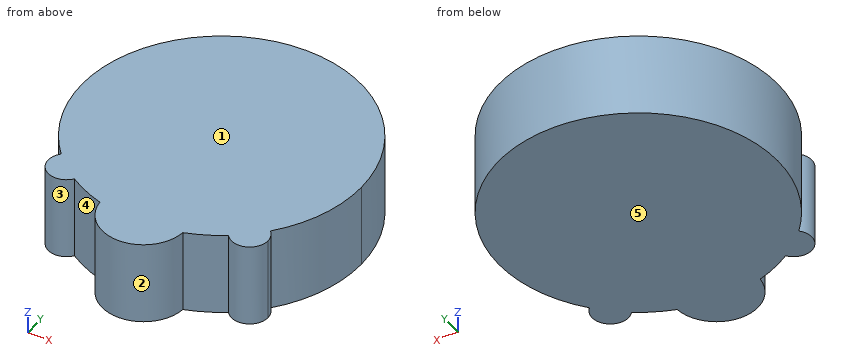
```python
from build123d import *

# Parameters (mm, degrees)
F1_DEPTH = 25


with BuildPart() as f1:
    # F0 (on Top) → F1 (new body)
    with BuildSketch(Plane.XY):
        with BuildLine():
            ThreePointArc((31.4123807864, -27.8794249104), (39.2639783582, -14.9110698304), (42, 0))
            ThreePointArc((42, 0), (-14.9110698304, 39.2639783582), (-31.4123807864, -27.8794249104))
            ThreePointArc((-31.4123807864, -27.8794249104), (-25.4105137384, -26.6574416615), (-22, -31.7450783587))
            ThreePointArc((-22, -31.7450783587), (-22.2864690998, -33.4969617889), (-23.1160347465, -35.066350503))
            ThreePointArc((-23.1160347465, -35.066350503), (-17.9613012827, -37.9656641748), (-12.4504239602, -40.1121794872))
            ThreePointArc((-12.4504239602, -40.1121794872), (-0.5566419395, -26.5124001605), (12.5, -39))
            ThreePointArc((12.5, -39), (12.4875998395, -39.5566419395), (12.4504239602, -40.1121794872))
            ThreePointArc((12.4504239602, -40.1121794872), (17.9613012827, -37.9656641748), (23.1160347465, -35.066350503))
            ThreePointArc((23.1160347465, -35.066350503), (23.8988095238, -27.5879847641), (31.4123807864, -27.8794249104))
        make_face()
        with BuildLine():
            ThreePointArc((-22, -31.7450783587), (-25.4105137384, -26.6574416615), (-31.4123807864, -27.8794249104))
            ThreePointArc((-31.4123807864, -27.8794249104), (-27.5, -31.7450783587), (-23.1160347465, -35.066350503))
            ThreePointArc((-23.1160347465, -35.066350503), (-22.2864690998, -33.4969617889), (-22, -31.7450783587))
        make_face()
        with BuildLine():
            ThreePointArc((-23.1160347465, -35.066350503), (-27.5, -31.7450783587), (-31.4123807864, -27.8794249104))
            ThreePointArc((-31.4123807864, -27.8794249104), (-31.1011904762, -35.9021719533), (-23.1160347465, -35.066350503))
        make_face()
        with BuildLine():
            ThreePointArc((33, -31.7450783587), (32.5876366972, -29.6555920971), (31.4123807864, -27.8794249104))
            ThreePointArc((31.4123807864, -27.8794249104), (27.5, -31.7450783587), (23.1160347465, -35.066350503))
            ThreePointArc((23.1160347465, -35.066350503), (29.2518834302, -36.9586092589), (33, -31.7450783587))
        make_face()
        with BuildLine():
            ThreePointArc((23.1160347465, -35.066350503), (27.5, -31.7450783587), (31.4123807864, -27.8794249104))
            ThreePointArc((31.4123807864, -27.8794249104), (23.8988095238, -27.5879847641), (23.1160347465, -35.066350503))
        make_face()
        with BuildLine():
            ThreePointArc((12.5, -39), (-0.5566419395, -26.5124001605), (-12.4504239602, -40.1121794872))
            ThreePointArc((-12.4504239602, -40.1121794872), (0, -42), (12.4504239602, -40.1121794872))
            ThreePointArc((12.4504239602, -40.1121794872), (12.4875998395, -39.5566419395), (12.5, -39))
        make_face()
        with BuildLine():
            ThreePointArc((12.4504239602, -40.1121794872), (0, -42), (-12.4504239602, -40.1121794872))
            ThreePointArc((-12.4504239602, -40.1121794872), (0, -51.5), (12.4504239602, -40.1121794872))
        make_face()
    extrude(amount=F1_DEPTH)


solid = f1.part
```
Source: CAD feature listing. Evaluate the final solid. Frame: model axes, mm. Face numbers are marked on the shaded views. A direction names the side the tool comes from. Round coordinates to 2 decimals unless told otherwise and drop trailing zeros. Write each loop counter-clockwise with the first axis right and the second up, starting at its lowest first coordinate (ties: lowest second). Pieces come first, ordered by that corner, then holes. Notation, with made-up numbers: M 5.25,17.25 L 18.25,17.25 A30 ccw 18.25,52.25 Z; hole C 84,-27.75 d2. An arc over 180 degrees is marked long. Answer as a JSON object with one key per item and string values. Group by question number.
(1) Section query B-B on x = 35. Output: boundary loops of the cut face in (y, z).
(2) First-contact query: pin 1 (2 mm diameter, centred on x = -4, y = -37.5, fed in from -Z); pin 2 (1 mm diameter, centred on y = 5, z = 16.5, fed in from +X); pin 3 (1.5 mm diameter, centred on y = -30, z = 9.5, fed in from -X); pin 4 (6 mm diameter, centred on x = -6.5, z = 6.5, fed in from -Y). Flat tips, straight axial feed; report the tip coordinate or a pass-through.
(3) Mould query, pull axis X, two halves, no side actions, for the marked faces 1, 2 and 3. Classes: +X half, -X half, draft (parallel to the pull), parting line (faces both ways), or undercut.
(4) Section query C-C on y = 13.5. Output: boundary loops of the cut face in (x, z), then the cut area to 3 significant figures.
(5) Section query A-A on z = 21.25. Output: boundary loops of the cut face in (x, y), then the cut area to 3 significant figures.
(6) Ray query, line 1 (X direction, y = -35.5, z = 1.5); line 2 (X direction, y = 19.5, z = 18.75); line 3 (Y direction, x = -13, z = 3.25). Return the intervals inside material, ascending. Write a range as [from, to].
(7) Reachability of the marked faces 4 and 5 from +Z, -Z, +X, -X, +Y, -Y: full face, straight path, thin tool, end or side. Return the list, or none.
Computed values:
{
 "1": {"outline": "M -23.22,0 L 23.22,0 L 23.22,25 L -23.22,25 Z"},
 "2": {"pin 1": "z = 0", "pin 2": "x = 41.76", "pin 3": "x = -32.91", "pin 4": "y = -51"},
 "3": {"face 1": "draft", "face 2": "parting line", "face 3": "undercut"},
 "4": {"outline": "M -39.77,0 L 39.77,0 L 39.77,25 L -39.77,25 Z", "area": "1,990 mm^2"},
 "5": {"outline": "M -31.41,-27.88 A5.5 ccw long -23.12,-35.07 A42 ccw -12.45,-40.11 A12.5 ccw 12.45,-40.11 A42 ccw 23.12,-35.07 A5.5 ccw long 31.41,-27.88 A42 ccw long Z", "area": "5,830 mm^2"},
 "6": {"line 1": "[-31.52, -23.48], [-22.44, 22.44], [23.48, 31.52]", "line 2": "[-37.2, 37.2]", "line 3": "[-39.94, 39.94]"},
 "7": {"face 4": "+Z, -Z, -Y", "face 5": "-Z, +X, -X, +Y, -Y"}
}
